from build123d import *

# Parameters (mm, degrees)
F0_R     = 11.125
F1_DEPTH = 7


with BuildPart() as f1:
    # F0 (on Top) → F1 (new body)
    with BuildSketch(Plane.XY):
        with BuildLine():
            Line((-14.270237, 23.338111), (-9.655566, 15.673587))
            ThreePointArc((-9.655566, 15.673587), (-8.967214, 12.565001), (-10.294885, 9.671141))
            ThreePointArc((-10.294885, 9.671141), (-12.217419, 7.088744), (-13.505254, 4.138083))
            ThreePointArc((-13.505254, 4.138083), (-15.276242, 1.610135), (-18.19413, 0.603733))
            Line((-18.19413, 0.603733), (-27.80012, 0.427443))
            Line((-27.80012, 0.427443), (-34.708436, -12.061889))
            Line((-34.708436, -12.061889), (-27.346516, -24.289332))
            Line((-27.346516, -24.289332), (-13.076279, -24.027443))
            Line((-13.076279, -24.027443), (-8.745941, -16.198759))
            ThreePointArc((-8.745941, -16.198759), (-6.398003, -14.048335), (-3.228012, -13.751202))
            ThreePointArc((-3.228012, -13.751202), (-0.030322, -14.124967), (3.168942, -13.764935))
            ThreePointArc((3.168942, -13.764935), (6.243703, -14.034681), (8.574217, -16.058446))
            Line((8.574217, -16.058446), (13.529883, -24.289332))
            Line((13.529883, -24.289332), (27.80012, -24.027443))
            Line((27.80012, -24.027443), (34.708436, -11.538111))
            Line((34.708436, -11.538111), (27.346516, 0.689332))
            Line((27.346516, 0.689332), (18.401507, 0.525172))
            ThreePointArc((18.401507, 0.525172), (15.365217, 1.483334), (13.522896, 4.080061))
            ThreePointArc((13.522896, 4.080061), (12.247742, 7.036224), (10.336312, 9.626852))
            ThreePointArc((10.336312, 9.626852), (9.032538, 12.424546), (9.619913, 15.454712))
            Line((9.619913, 15.454712), (14.270237, 23.861889))
            Line((14.270237, 23.861889), (6.908316, 36.089332))
            Line((6.908316, 36.089332), (-7.361921, 35.827443))
            Line((-7.361921, 35.827443), (-14.270237, 23.338111))
        make_face()
        Polygon((-26.285783, -2.087725), (-14.950914, -1.879706), (-9.103331, -11.591982), (-14.590616, -21.512275), (-25.925485, -21.720294), (-31.773068, -12.008018), align=None, mode=Mode.SUBTRACT)
        Polygon((14.950914, -21.720294), (9.103331, -12.008018), (14.590616, -2.087725), (25.925485, -1.879706), (31.773068, -11.591982), (26.285783, -21.512275), align=None, mode=Mode.SUBTRACT)
        Circle(F0_R, mode=Mode.SUBTRACT)
        Polygon((-5.487285, 13.679706), (-11.334869, 23.391982), (-5.847584, 33.312275), (5.487285, 33.520294), (11.334869, 23.808018), (5.847584, 13.887725), align=None, mode=Mode.SUBTRACT)
    extrude(amount=F1_DEPTH)


solid = f1.part
Could you check a few things on this model? Use its own coordinates, in mm. A direction names the side the tool comes from. Coordinates: 2 decimals unless noted, no trailing zeros. Order: outer loops, then holes, each group sorted by start corner. A loop starts at its lowest first (then second) coordinate and runs counter-clockwise, first axis right, second up. Notation, with made-up numbers: (30, 87.25) - (75, 87.25) arc R29 cw to (75, 118.25) - close; hole circle Ø4 at (30.5, -15.5). An arc over 180 degrees is marked (long way). Answer in a Markdown table with one row per item. Add a question column.
(1) If we section it at D-D, the plane z = 2.75: State how many separate pieces and enclosed holes the cut face has, then the cut area to 3 significant figures.
(2) If we mould it in two halves opening along X, with no side actions, what happens to faces 3 (the face through (10, 6, 0)), 4 (the face through (-8.2, 7.52, 3.45)), 5 (the face through (11.913, 19.599, 3.451))? For each: released by +X, released by -X, zero draft, split by the parting line, or undercut.
(3) If we section it at A-A, the plane x = -2: Please give me the cut outline in (y, z).
(4) Will these pins go through, and if not, where does the flat tip stop? pin 1 (3 mm diameter, centred on x = -13, z = 2.5, fed in from +Y); pin 2 (4 mm diameter, centred on x = 22, z = 2.5, fed in from -Y); pin 3 (1 mm diameter, centred on y = -13.5, z = 6, fed in from -X).
(5) If we section it at C-C, the plane y = 7: Please give me the cut outline in (x, z).
(6) If we section it at B-B, the plane y = -5: Please give me the cut outline in (x, z), then the cut area to 3 significant figures.
(7) I need wall thicknesses on L1, parallel to Y at x = 0, z = 3.5 (3 decimals); L2, parallel to Y at x = -3.5, z = 0.75; L3, parallel to X at y = -17, z = 2. Which ranges of each line are inside material? Lowest first, please.
(8) On a 3-axis mill with a long thin cutter (end or side, diameter ignored), from which of +Z, -Z, +X, -X, +Y, -Y can I reach the whole of each face in a straight line? I mean faces 1 (the face through (-12.068, -6.668, 3.451)), 2 (the face through (-10.77, 29.67, 3.45)). Say none if no direction works.
Results are:
| question | item | result |
|---|---|---|
| 1 | separate pieces | 1 |
| 1 | enclosed holes | 4 |
| 1 | area | 745 mm2 |
| 2 | face 3 | zero draft |
| 2 | face 4 | undercut |
| 2 | face 5 | released by +X |
| 3 | outline | (-13.98, 0) - (-10.94, 0) - (-10.94, 7) - (-13.98, 7) - close; (10.94, 0) - (13.74, 0) - (13.74, 7) - (10.94, 7) - close; (33.38, 0) - (35.93, 0) - (35.93, 7) - (33.38, 7) - close |
| 4 | pin 1 | stops at y = 28.35 |
| 4 | pin 2 | stops at y = -24.17 |
| 4 | pin 3 | stops at x = -34.14 |
| 5 | outline | (-12.27, 0) - (-8.65, 0) - (-8.65, 7) - (-12.27, 7) - close; (8.65, 0) - (12.27, 0) - (12.27, 7) - (8.65, 7) - close |
| 6 | outline | (-30.8, 0) - (-27.9, 0) - (-27.9, 7) - (-30.8, 7) - close; (-13.07, 0) - (-9.94, 0) - (-9.94, 7) - (-13.07, 7) - close; (9.94, 0) - (12.98, 0) - (12.98, 7) - (9.94, 7) - close; (27.8, 0) - (30.77, 0) - (30.77, 7) - (27.8, 7) - close |
| 6 | area | 84.3 mm2 |
| 7 | L1 | y = -14.125 to -11.125, 11.125 to 13.78, 33.42 to 35.963 |
| 7 | L2 | y = -13.7 to -10.56, 10.56 to 13.72, 33.36 to 35.9 |
| 7 | L3 | x = -31.74 to -28.77, -12.09 to -9.19, 9.14 to 12.11, 28.78 to 31.69 |
| 8 | face 1 | +Z, -Z |
| 8 | face 2 | +Z, -Z, -X, +Y |
